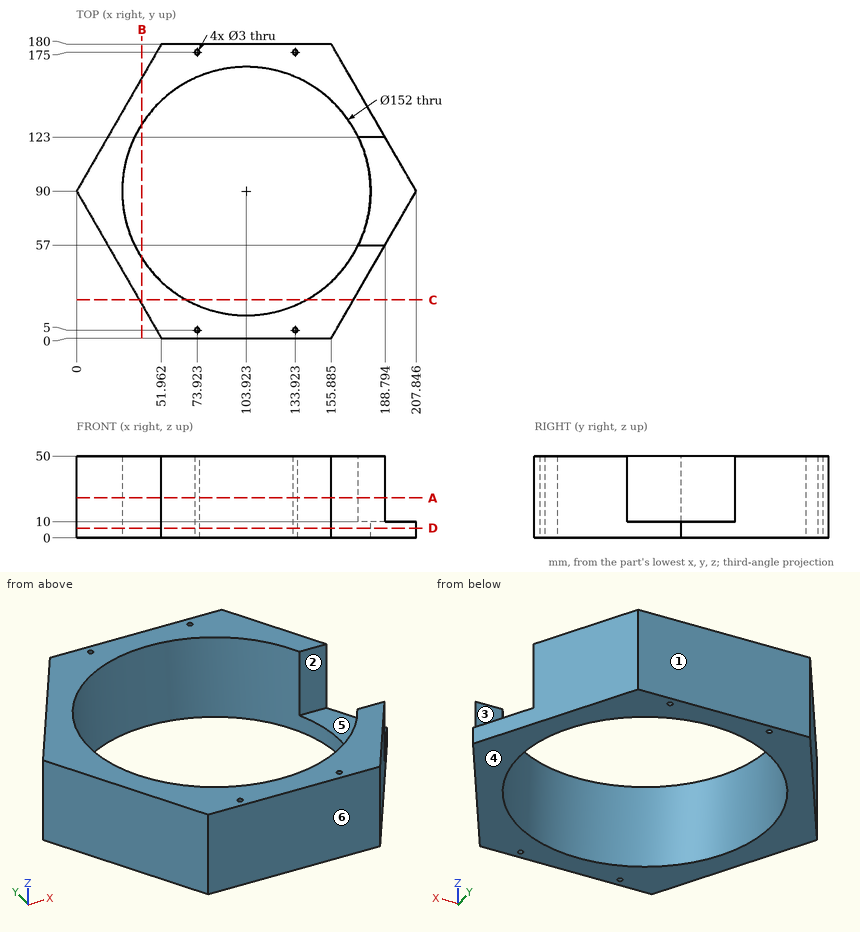
Drawing for the job (mm, zero at the part's lowest x, y, z). A direction names the side the tool comes from. Give positions to 0.01 mm unless a question says otherwise; leave off trailing zeros. Loops run counter-clockwise (first coordinate to the right, second up) from the corner with the lowest first, then second, coordinate; pieces in that order, holes last.
1) Band-saw the part on B-B on x = 40. List the corners of the cut face in (y, z).
Values follow:
outline: (20.72, 0) - (48.89, 0) - (48.89, 50) - (20.72, 50) - close; (131.11, 0) - (159.28, 0) - (159.28, 50) - (131.11, 50) - close
2) 3-axis set-ups, long thin cutter, end or side, ignore diameter. For the marked faces 1 and 2: which of +Z, -Z, +X, -X, +Y, -Y reach the whole face in a straight line?
Values follow:
face 1: +Z, -Z, +X, -X, +Y
face 2: +Z, +X
3) Probe line 1 along X through (y, z) = (5, 25) (1 decimal); line 2 along Y through (x, z) = (110, 10.5); line 3 along X through (y, z) = (36.5, 32.5) (1 decimal). List the from-to ranges inside material, lowest first.
Values follow:
line 1: x = 49.1 to 72.4, 75.4 to 132.4, 135.4 to 158.8
line 2: y = 0 to 14.24, 165.76 to 180
line 3: x = 30.9 to 49.9, 157.9 to 177
4) Band-saw the part on A-A on z = 24.5. List the corners of the cut face in (x, y) (1 decimal), then the cut area to 3 significant figures.
Values follow:
outline: (0, 90) - (52, 0) - (155.9, 0) - (188.8, 57) - (172.4, 57) arc R76 cw (long way) to (172.4, 123) - (188.8, 123) - (155.9, 180) - (52, 180) - close; hole circle Ø3 at (73.9, 5); hole circle Ø3 at (73.9, 175); hole circle Ø3 at (133.9, 5); hole circle Ø3 at (133.9, 175)
area: 8,510 mm2
5) Two-plate mould, pull along Y, no slides. Class the marked faces 3, 4, 5 and 6: released by +Y, released by -Y, zero draft, split by the parting line, or undercut.
Values follow:
face 3: undercut
face 4: zero draft
face 5: undercut
face 6: released by -Y
6) Band-saw the part on D-D on z = 6. List the corners of the cut face in (x, y) (1 decimal).
Values follow:
outline: (0, 90) - (52, 0) - (155.9, 0) - (207.8, 90) - (155.9, 180) - (52, 180) - close; hole circle Ø152 at (103.9, 90); hole circle Ø3 at (73.9, 5); hole circle Ø3 at (73.9, 175); hole circle Ø3 at (133.9, 5); hole circle Ø3 at (133.9, 175)
7) Drop flat-ended pins along their axis: P1, Ø10.5, axis at x = 198, y = 96, coming from the +Z side; P2, Ø5, axis at x = 177.5, z = 26, coming from the +Y side; P3, Ø4, axis at y = 73, z = 30, coming from the +X side. Give the stop position or say it passes through.
Values follow:
P1: stops at z = 10
P2: stops at y = 146.89
P3: stops at x = 30.34
8) Band-saw the part on C-C on y = 23.5. List the corners of the cut face in (x, z).
Values follow:
outline: (38.39, 0) - (67.13, 0) - (67.13, 50) - (38.39, 50) - close; (140.72, 0) - (169.45, 0) - (169.45, 50) - (140.72, 50) - close
